Part model, mm, in its own coordinate system. Face numbers are marked on the shaded views. A direction names the side the tool comes from. Coordinates: 2 decimals unless noted, no trailing zeros. Order: outer loops, then holes, each group sorted by start corner. A loop starts at its lowest first (then second) coordinate and runs counter-clockwise, first axis right, second up.
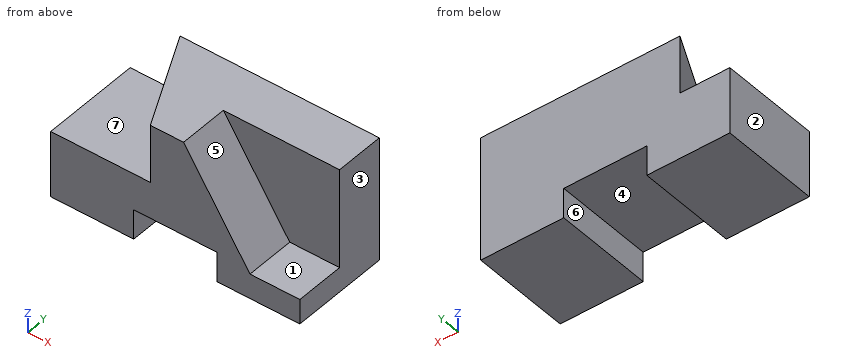
from build123d import *

# Parameters (mm, degrees)
F1_DEPTH = 60
F3_DEPTH = 30
F5_DEPTH = 35


with BuildPart() as f1:
    # F0 (on Front) → F1 (new body)
    with BuildSketch(Plane.XZ):
        Polygon((-75, 40), (-75, 0), (-25, 0), (-25, 18), (25, 18), (25, 0), (75, 0), (75, 75), (-45, 75), (-45, 40), align=None)
    extrude(amount=F1_DEPTH)

    # F2 (on face) → F3 (cut)
    with BuildSketch(Plane.XZ.offset(60)):
        Polygon((75, 15), (75, 75), (5, 75), (45, 15), align=None)
    extrude(amount=-F3_DEPTH, mode=Mode.SUBTRACT)

    # F4 (on face) → F5 (cut)
    with BuildSketch(Plane.XY.offset(75)):
        Polygon((-15, -60), (-45, 0), (-45, -60), align=None)
    extrude(amount=-F5_DEPTH, mode=Mode.SUBTRACT)


solid = f1.part
Q1. Cut at D-D on y = -18. Write the cut outline in (x, z), and give its area (4 significant figures).
Results list:
outline: (-75, 0) - (-25, 0) - (-25, 18) - (25, 18) - (25, 0) - (75, 0) - (75, 75) - (-36, 75) - (-36, 40) - (-75, 40) - close
area: 8,985 mm2
Q2. Cut at C-C on z = 34. Write the cut outline in (x, y), and give its area (3 significant figures).
Results list:
outline: (-75, -60) - (32.33, -60) - (32.33, -30) - (75, -30) - (75, 0) - (-75, 0) - close
area: 7,720 mm2
Q3. Cut at B-B on x = 27.5. Write the cut outline in (y, z).
Results list:
outline: (-60, 0) - (0, 0) - (0, 75) - (-30, 75) - (-30, 41.25) - (-60, 41.25) - close
Q4. Mould opens along X. For the marked faces 1, 2, 3 and 4 say: pulls with the +X half, pulls with the -X half, needs draft (parallel to the pull), parting line crosses it, or undercut.
Results list:
face 1: needs draft
face 2: pulls with the -X half
face 3: pulls with the +X half
face 4: undercut
Q5. Wall check: line 1 along X through (y, z) = (-25, 4); line 2 along Z through (x, y) = (-56, -7.5); line 3 along Z through (x, y) = (-18.5, -47). Give the ranges that are in metal, low to high.
Results list:
line 1: x = -75 to -25, 25 to 75
line 2: z = 0 to 40
line 3: z = 18 to 75
Q6. Which spindle directions (+Z, -Z, +X, -X, +Y, -Y) get a long thin tool onto all of the face, cutting with end or side? Do the marked faces 5, 6 and 7. Say none if no direction does.
Results list:
face 5: +Z, +X, -Y
face 6: -Z, +Y, -Y
face 7: +Z, -X, -Y
Q7. Pin check, flat tips, straight feed: pin 1 Ø2 at (x, z) = (47, 34.5) entering from -Y; pin 2 Ø1.5 at (x, z) = (-28, 48) entering from +Y; pin 3 Ø15 at (x, y) = (-6, -40.5) entering from -Z. Stop position of each tip, or through.
Results list:
pin 1: stops at y = -30
pin 2: stops at y = 0
pin 3: stops at z = 18
Q8. Cut at A-A on y = -34.5. Write the cut outline in (x, z).
Results list:
outline: (-75, 0) - (-25, 0) - (-25, 18) - (25, 18) - (25, 0) - (75, 0) - (75, 15) - (45, 15) - (5, 75) - (-27.75, 75) - (-27.75, 40) - (-75, 40) - close
